from build123d import *

# Parameters (mm, degrees)
SKETCH_1_W          = 20
SKETCH_1_H          = 20
SKETCH_1_W_2        = 17
SKETCH_1_H_2        = 17
EXTRUDE_1_DEPTH     = 680
CUT_EXTRUDE_1_DEPTH = 681.367547727


with BuildPart() as part:
    # ｽｹｯﾁ1 → ﾎﾞｽ - 押し出し1 (new body)
    with BuildSketch(Plane.XY):
        Rectangle(SKETCH_1_W, SKETCH_1_H)
        Rectangle(SKETCH_1_W_2, SKETCH_1_H_2, mode=Mode.SUBTRACT)
    extrude(amount=EXTRUDE_1_DEPTH)

    # ｽｹｯﾁ2 → ｶｯﾄ - 押し出し1 (cut, through all)
    with BuildSketch(Plane.ZY.offset(10)):
        with BuildLine():
            Line((660, -4), (630, -4))
            ThreePointArc((630, -4), (626, 0), (630, 4))
            Line((630, 4), (660, 4))
            ThreePointArc((660, 4), (664, 0), (660, -4))
        make_face()
        with BuildLine():
            Line((20, -4), (50, -4))
            ThreePointArc((50, -4), (54, 0), (50, 4))
            Line((50, 4), (20, 4))
            ThreePointArc((20, 4), (16, 0), (20, -4))
        make_face()
    extrude(amount=-CUT_EXTRUDE_1_DEPTH, mode=Mode.SUBTRACT)


solid = part.part
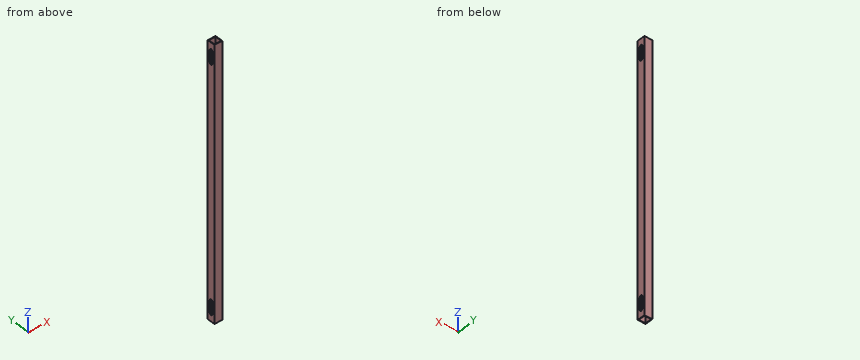
The listing builds one solid part. Answer for the finished solid, in the listing's coordinates (mm). Coordinates: 2 decimals unless noted, no trailing zeros. Write each loop counter-clockwise with the first axis right and the second up, starting at its lowest first coordinate (ties: lowest second). Pieces come first, ordered by that corner, then holes. Notation, with made-up numbers: M -16,-18.5 L 17,-18.5 A14 cw 17,0.5 Z; hole C -3.75,25 d3. An arc over 180 degrees is marked long. Put each result on its own line as item: value. Start each with the question number.
1. Consider line 1 (Y direction, x = -5.5, z = 139.5). Determine where the line is inside the solid, lowest interval first. Write a range as from..to.
2. A cutting plane is placed at A-A on x = -3. Write down the section's boundary in (y, z), then the cut area to 3 significant figures.
3. A cutting plane is placed at B-B on y = 0. Write down the section's boundary in (x, z), then the cut area to 3 significant figures.
4. A cutting plane is placed at C-C on z = 90.5. Write down the section's boundary in (x, y), then the cut area to 3 significant figures.
Resolved:
1. line 1: y = -10..-8.5, 8.5..10
2. outline: M -10,0 L -8.5,0 L -8.5,680 L -10,680 Z; M 8.5,0 L 10,0 L 10,680 L 8.5,680 Z
2. area: 2,040 mm2
3. outline: M -10,0 L -8.5,0 L -8.5,16 L -10,16 Z; M -10,54 L -8.5,54 L -8.5,626 L -10,626 Z; M -10,664 L -8.5,664 L -8.5,680 L -10,680 Z; M 8.5,0 L 10,0 L 10,16 L 8.5,16 Z; M 8.5,54 L 10,54 L 10,626 L 8.5,626 Z; M 8.5,664 L 10,664 L 10,680 L 8.5,680 Z
3. area: 1,810 mm2
4. outline: M -10,-10 L 10,-10 L 10,10 L -10,10 Z; hole M -8.5,-8.5 L 8.5,-8.5 L 8.5,8.5 L -8.5,8.5 Z
4. area: 111 mm2
